Build history of the part. All positions in model axes, mm. Round coordinates to 2 decimals unless told otherwise and drop trailing zeros. Write each loop counter-clockwise with the first axis right and the second up, starting at its lowest first coordinate (ties: lowest second). Pieces come first, ordered by that corner, then holes.
from build123d import *

# Parameters (mm, degrees)
F0_R     = 26.761417
F0_R_2   = 4.9
F0_R_3   = 11.3
F1_DEPTH = 8
F2_R     = 2


with BuildPart() as f1:
    # F0 (on Top) → F1 (new body)
    with BuildSketch(Plane.XY):
        Circle(F0_R)
        with Locations((-16.497784, -9.525)):
            Circle(F0_R_2, mode=Mode.SUBTRACT)
        with Locations((0, -19.05)):
            Circle(F0_R_2, mode=Mode.SUBTRACT)
        with Locations((16.497784, -9.525)):
            Circle(F0_R_2, mode=Mode.SUBTRACT)
        with Locations((-16.497784, 9.525)):
            Circle(F0_R_2, mode=Mode.SUBTRACT)
        Circle(F0_R_3, mode=Mode.SUBTRACT)
        with Locations((16.497784, 9.525)):
            Circle(F0_R_2, mode=Mode.SUBTRACT)
        with Locations((0, 19.05)):
            Circle(F0_R_2, mode=Mode.SUBTRACT)
    extrude(amount=F1_DEPTH)

    # F2
    f2_edges = [f1.edges().sort_by_distance(p)[0] for p in [
        (-11.3, 0, 8),
        (-11.3, 0, 0),
        (-26.761417, 0, 0),
        (-26.761417, 0, 8),
    ]]
    fillet(f2_edges, radius=F2_R)


solid = f1.part
1) Mould opens along Y. For faces 1 (the cylindrical face through (-5.801, -26.125, 3.972)), 2 (the cylindrical face through (10.78, 3.39, 3.97)), 3 (the flat face through (11, -11, 8)) say: released by +Y, released by -Y, zero draft, split by the parting line, or undercut.
Results:
face 1: split by the parting line
face 2: undercut
face 3: zero draft
2) Slice it at B-B (x = 0). Write the cut outline in (y, z), plus the area to 3 significant figures.
Results:
outline: (-26.76, 2) arc R2 ccw to (-24.76, 0) - (-23.95, 0) - (-23.95, 8) - (-24.76, 8) arc R2 ccw to (-26.76, 6) - close; (-14.15, 0) - (-13.3, 0) arc R2 ccw to (-11.3, 2) - (-11.3, 6) arc R2 ccw to (-13.3, 8) - (-14.15, 8) - close; (11.3, 2) arc R2 ccw to (13.3, 0) - (14.15, 0) - (14.15, 8) - (13.3, 8) arc R2 ccw to (11.3, 6) - close; (23.95, 0) - (24.76, 0) arc R2 ccw to (26.76, 2) - (26.76, 6) arc R2 ccw to (24.76, 8) - (23.95, 8) - close
area: 83.7 mm2
3) Pin check, flat tips, straight feed: pin 1 Ø1.5 at (x, z) = (11.5, 3) entering from -Y; pin 2 Ø1.5 at (y, z) = (-14.5, 6.5) entering from -X. Stop position of each tip, or through.
Results:
pin 1: stops at y = -24.51
pin 2: stops at x = -22.92
4) Wall check: L1, parallel to Y at x = 0, z = 5.5; L2, parallel to Y at x = -12, z = 6.25; L3, parallel to Y at x = 18.5, z = 4.5. Give the ranges that are in metal, low to high.
Results:
L1: y = -26.76 to -23.95, -14.15 to -11.3, 11.3 to 14.15, 23.95 to 26.76
L2: y = -23.9 to -11.47, -7.58 to 7.58, 11.47 to 23.9
L3: y = -19.34 to -14, -5.05 to 5.05, 14 to 19.34
5) Slice it at A-A (y = 0). Write the cut outline in (x, z), plus the area to 3 significant figures.
Results:
outline: (-26.76, 2) arc R2 ccw to (-24.76, 0) - (-13.3, 0) arc R2 ccw to (-11.3, 2) - (-11.3, 6) arc R2 ccw to (-13.3, 8) - (-24.76, 8) arc R2 ccw to (-26.76, 6) - close; (11.3, 2) arc R2 ccw to (13.3, 0) - (24.76, 0) arc R2 ccw to (26.76, 2) - (26.76, 6) arc R2 ccw to (24.76, 8) - (13.3, 8) arc R2 ccw to (11.3, 6) - close
area: 241 mm2
6) Slice it at C-C (z = 1). Write the cut outline in (x, y) (3 decimals), plus the area to 3 significant figures.
Results:
outline: circle Ø52.987 at (0, 0); hole circle Ø9.8 at (-16.498, -9.525); hole circle Ø9.8 at (-16.498, 9.525); hole circle Ø23.136 at (0, 0); hole circle Ø9.8 at (0, -19.05); hole circle Ø9.8 at (0, 19.05); hole circle Ø9.8 at (16.498, -9.525); hole circle Ø9.8 at (16.498, 9.525)
area: 1,330 mm2
